from build123d import *

# Parameters (mm, degrees)
SKETCH2_R           = 6.35
BOSS_EXTRUDE1_DEPTH = 31.75
SKETCH8_R           = 6.35
BOSS_EXTRUDE2_DEPTH = 31.75


with BuildPart() as part:
    # Sketch2 → Boss-Extrude1 (new body)
    with BuildSketch(Plane.XY):
        Circle(SKETCH2_R)
    extrude(amount=BOSS_EXTRUDE1_DEPTH)

    # Sketch7 → Revolve1 (revolve)
    with BuildSketch(Plane(origin=(0, 0, 0), x_dir=(0, 0, -1), z_dir=(1, 0, 0)), mode=Mode.PRIVATE) as revolve1_sk:
        with BuildLine():
            Line((-69.85, 0), (-50.8, 0))
            Line((-50.8, 0), (-50.8, 4.03225))
            ThreePointArc((-50.8, 4.03225), (-60.39523925, 4.613816096), (-69.85, 6.35))
            Line((-69.85, 6.35), (-69.85, 0))
        make_face()
        with BuildLine():
            Line((-50.8, 0), (-31.75, 0))
            Line((-31.75, 0), (-31.75, 6.35))
            ThreePointArc((-31.75, 6.35), (-41.20476075, 4.613816096), (-50.8, 4.03225))
            Line((-50.8, 4.03225), (-50.8, 0))
        make_face()
    revolve(revolve1_sk.sketch.rotate(Axis((0, 0, 0), (0, 0, 1)), 90), axis=Axis((0, 0, 0), (0, 0, 1)))

    # Sketch8 → Boss-Extrude2 (add)
    with BuildSketch(Plane.XY.offset(69.85)):
        Circle(SKETCH8_R)
    extrude(amount=BOSS_EXTRUDE2_DEPTH)


solid = part.part
Work out the finished part from the listing and answer in its coordinate system (mm). Round coordinates to 2 decimals unless told otherwise and drop trailing zeros. Write each loop counter-clockwise with the first axis right and the second up, starting at its lowest first coordinate (ties: lowest second). Pieces come first, ordered by that corner, then holes. Notation, with made-up numbers: (-30.5, 27) - (-21.5, 27) arc R12 cw to (-21.5, 43) - close; hole circle Ø5 at (52, 31.5). An arc over 180 degrees is marked (long way). Answer in a Markdown table with one row per item. Add a question column.
1. A cutting plane is placed at A-A, the plane z = 17. Determine the outline of the cut face in (x, y).
2. Given pin 1 (2 mm diameter, centred on x = 1.5, z = 61.5, fed in from -Y); pin 2 (6 mm diameter, centred on x = -2.5, z = 51.5, fed in from -Y); pin 3 (1 mm diameter, centred on x = -4, z = 28.5, fed in from +Y); pin 4 (2 mm diameter, centred on x = -5, y = 2.5, fed in from -Z), each flat-ended and moving along its own axis, determine where each tip first touches the part or whether it passes through.
3. A cutting plane is placed at B-B, the plane z = 65.5. Determine the outline of the cut face in (x, y).
4. Find the intervals of material crossed by line 1 along Y through (x, z) = (5.75, 82); line 2 along Y through (x, z) = (-3.25, 11); line 3 along X through (y, z) = (2.75, 19.5), in increasing order. Write a range as from..to.
Worked out:
| question | item | result |
|---|---|---|
| 1 | outline | circle Ø12.7 at (0, 0) |
| 2 | pin 1 | y = -4.79 |
| 2 | pin 2 | y = -4.07 |
| 2 | pin 3 | y = 5.3 |
| 2 | pin 4 | z = 0 |
| 3 | outline | circle Ø10.81 at (0, 0) |
| 4 | line 1 | -2.69..2.69 |
| 4 | line 2 | -5.46..5.46 |
| 4 | line 3 | -5.72..5.72 |
